Answer from the drawing. Dimensions are ordinates in mm from the lowest x, y and z of the part. A direction names the side the tool comes from. Give positions to 0.01 mm unless a question says otherwise; leave off trailing zeros. Order: outer loops, then holes, each group sorted by start corner. A loop starts at its lowest first (then second) coordinate and runs counter-clockwise, first axis right, second up.
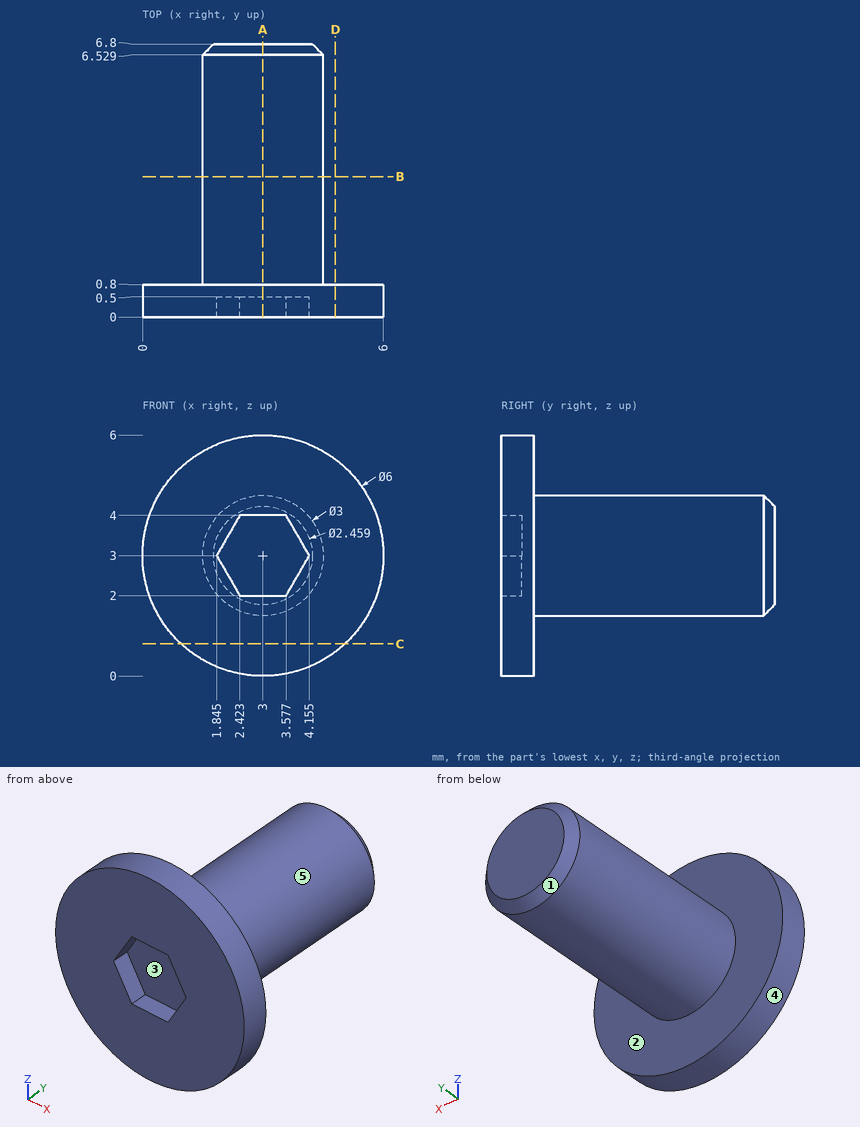
1. The part is cut by section C-C (z = 0.8). Write down the section's boundary in (x, y).
Findings below:
outline: (0.96, 0) - (5.04, 0) - (5.04, 0.8) - (0.96, 0.8) - close
2. Which of the six approach directions +Z, -Z, +X, -X, +Y, -Y give full straight-line access (tool end or side, diameter ignored) to the marked faces 4 and 5?
Findings below:
face 4: +Y, -Y
face 5: +Y
3. The mould has two halves that part along Z. Classify the marked faces 1, 2 and 3: pulls with the +Z half, pulls with the -Z half, needs draft (parallel to the pull), parting line crosses it, or undercut.
Findings below:
face 1: parting line crosses it
face 2: needs draft
face 3: undercut
4. The part is cut by section A-A (x = 3). Write down the section's boundary in (y, z).
Findings below:
outline: (0, 0) - (0.8, 0) - (0.8, 1.5) - (6.53, 1.5) - (6.8, 1.77) - (6.8, 4.23) - (6.53, 4.5) - (0.8, 4.5) - (0.8, 6) - (0, 6) - (0, 4) - (0.5, 4) - (0.5, 2) - (0, 2) - close
5. The part is cut by section D-D (x = 4.8). Write down the section's boundary in (y, z).
Findings below:
outline: (0, 0.6) - (0.8, 0.6) - (0.8, 5.4) - (0, 5.4) - close
6. Straight lines are drawn through the part: probe 1 along Y at (x, z) = (4.75, 4.1); probe 2 along Y at (x, z) = (3.2, 2.75); probe 3 along X at (y, z) = (2, 3.5) (1 decimal). For each, find the intervals that lie inside material, in ascending order.
Findings below:
probe 1: y = 0 to 0.8
probe 2: y = 0.5 to 6.8
probe 3: x = 1.6 to 4.4
7. The part is cut by section B-B (y = 3.5). Write down the section's boundary in (x, z).
Findings below:
outline: circle Ø3 at (3, 3)
